```python
from build123d import *

# Parameters (mm, degrees)
SKETCH1_W               = 449.58
SKETCH1_H               = 449.58
BOSS_EXTRUDE1_DEPTH     = 6.35
CUT_EXTRUDE1_DEPTH      = 318.964480249
CUT_EXTRUDE1_DEPTH_BACK = 318.964480249
SKETCH2_R               = 1.984375
SKETCH2_R_2             = 27.432
SKETCH3_W               = 9.5
SKETCH3_H               = 12
CUT_EXTRUDE2_DEPTH      = 318.964480249
SKETCH4_R               = 2.1828125
CUT_EXTRUDE3_DEPTH      = 318.964480249
SKETCH5_R               = 2.1828125
CUT_EXTRUDE4_DEPTH      = 318.964480249


with BuildPart() as part:
    # Sketch1 → Boss-Extrude1 (new body)
    with BuildSketch(Plane(origin=(0, 0, 0), x_dir=(1, 0, 0), z_dir=(0, 1, 0))):
        Rectangle(SKETCH1_W, SKETCH1_H)
    extrude(amount=BOSS_EXTRUDE1_DEPTH)

    # Sketch2 → Cut-Extrude1 (cut, two sides: drawn at the far end of the back side and taken through both)
    with BuildSketch(Plane(origin=(0, 6.35, 0), x_dir=(1, 0, 0), z_dir=(0, 1, 0)).offset(-CUT_EXTRUDE1_DEPTH_BACK)):
        with Locations(Location((-44.8437, 44.8437, 0), (0, 0, 270))):
            Circle(SKETCH2_R)
        with Locations(Location((44.8437, 44.8437, 0), (0, 0, 270))):
            Circle(SKETCH2_R)
        with Locations(Location((-44.8437, -44.8437, 0), (0, 0, 270))):
            Circle(SKETCH2_R)
        with Locations(Location((44.8437, -44.8437, 0), (0, 0, 270))):
            Circle(SKETCH2_R)
        with Locations(Location((0, 0, 0), (0, 0, 270))):
            Circle(SKETCH2_R_2)
    extrude(amount=CUT_EXTRUDE1_DEPTH + CUT_EXTRUDE1_DEPTH_BACK, mode=Mode.SUBTRACT)

    # Sketch3 → Cut-Extrude2 (cut, through all)
    with BuildSketch(Plane(origin=(0, 6.35, 0), x_dir=(1, 0, 0), z_dir=(0, 1, 0))):
        with Locations((168.828815076, -168.828815076)):
            Rectangle(SKETCH3_W, SKETCH3_H)
    extrude(amount=-CUT_EXTRUDE2_DEPTH, mode=Mode.SUBTRACT)

    # Sketch4 → Cut-Extrude3 (cut, through all)
    with BuildSketch(Plane(origin=(0, 6.35, 0), x_dir=(1, 0, 0), z_dir=(0, 1, 0))):
        with Locations(Location((-212.09, 212.09, 0), (0, 0, 270))):
            Circle(SKETCH4_R)
        with Locations(Location((-186.69, 212.09, 0), (0, 0, 270))):
            Circle(SKETCH4_R)
        with Locations(Location((-212.09, 186.69, 0), (0, 0, 270))):
            Circle(SKETCH4_R)
        with Locations(Location((-186.69, 186.69, 0), (0, 0, 270))):
            Circle(SKETCH4_R)
        with Locations(Location((186.69, 212.09, 0), (0, 0, 270))):
            Circle(SKETCH4_R)
        with Locations(Location((186.69, 186.69, 0), (0, 0, 270))):
            Circle(SKETCH4_R)
        with Locations(Location((212.09, 186.69, 0), (0, 0, 270))):
            Circle(SKETCH4_R)
        with Locations(Location((212.09, 212.09, 0), (0, 0, 270))):
            Circle(SKETCH4_R)
        with Locations(Location((186.69, -186.69, 0), (0, 0, 270))):
            Circle(SKETCH4_R)
        with Locations(Location((212.09, -186.69, 0), (0, 0, 270))):
            Circle(SKETCH4_R)
        with Locations(Location((212.09, -212.09, 0), (0, 0, 270))):
            Circle(SKETCH4_R)
        with Locations(Location((186.69, -212.09, 0), (0, 0, 270))):
            Circle(SKETCH4_R)
        with Locations(Location((-212.09, -186.69, 0), (0, 0, 270))):
            Circle(SKETCH4_R)
        with Locations(Location((-186.69, -186.69, 0), (0, 0, 270))):
            Circle(SKETCH4_R)
        with Locations(Location((-186.69, -212.09, 0), (0, 0, 270))):
            Circle(SKETCH4_R)
        with Locations(Location((-212.09, -212.09, 0), (0, 0, 270))):
            Circle(SKETCH4_R)
    extrude(amount=-CUT_EXTRUDE3_DEPTH, mode=Mode.SUBTRACT)

    # Sketch5 → Cut-Extrude4 (cut, through all)
    with BuildSketch(Plane(origin=(0, 6.35, 0), x_dir=(1, 0, 0), z_dir=(0, 1, 0))):
        with Locations(Location((-191.419449709, 134.033341647, 0), (0, 0, 270))):
            Circle(SKETCH5_R)
        with BuildLine():
            ThreePointArc((-121.64596733, 192.580244977), (-139.176494703, 208.644013705), (-160.267293124, 219.623188433))
            ThreePointArc((-160.267293124, 219.623188433), (-163.065031767, 218.318581478), (-161.760424812, 215.520842836))
            ThreePointArc((-161.760424812, 215.520842836), (-141.680514333, 205.067903062), (-124.990230102, 189.774075318))
            ThreePointArc((-124.990230102, 189.774075318), (-121.915013887, 189.505028762), (-121.64596733, 192.580244977))
        make_face()
    extrude(amount=-CUT_EXTRUDE4_DEPTH, mode=Mode.SUBTRACT)


solid = part.part
```
The model under review builds one solid part; all positions refer to its coordinate system, in mm. Round coordinates to 2 decimals unless told otherwise and drop trailing zeros. Order: outer loops, then holes, each group sorted by start corner. A loop starts at its lowest first (then second) coordinate and runs counter-clockwise, first axis right, second up. Notation, with made-up numbers: (72.5, 8.25) - (84.5, 8.25) arc R12 ccw to (84.5, 30.25) - close; hole circle Ø2 at (18, 58.25). An arc over 180 degrees is marked (long way). Answer in a Markdown table with one row per item.
(1) Take a section at A-A on x = 0. Write out the cut boundary in (y, z).
Result set:
| item | result |
|---|---|
| outline | (0, -224.79) - (6.35, -224.79) - (6.35, -27.43) - (0, -27.43) - close; (0, 27.43) - (6.35, 27.43) - (6.35, 224.79) - (0, 224.79) - close |
(2) Mouldability with a two-part tool opening along X and no side actions: class faces 1 (the face through (-3, 0, -53)), 2 (the face through (-141.94, 3.22, -205.25)), 3 (the face through (-138.9, 3.22, -208.45)) as released by +X, released by -X, zero draft, split by the parting line, or undercut.
Result set:
| item | result |
|---|---|
| face 1 | zero draft |
| face 2 | undercut |
| face 3 | undercut |
(3) Take a section at B-B on z = 0. Write out the cut boundary in (x, y).
Result set:
| item | result |
|---|---|
| outline | (-224.79, 0) - (-27.43, 0) - (-27.43, 6.35) - (-224.79, 6.35) - close; (27.43, 0) - (224.79, 0) - (224.79, 6.35) - (27.43, 6.35) - close |
(4) For line 1 (Z direction, x = -186.69, y = 5); line 2 (Z direction, x = -137, y = 5.25), list the stretches that pass through material, from the lowest coordinate up. Write a range as from..to.
Result set:
| item | result |
|---|---|
| line 1 | z = -224.79..-214.27, -209.91..-188.87, -184.51..184.51, 188.87..209.91, 214.27..224.79 |
| line 2 | z = -224.79..-207.07, -201.55..224.79 |
(5) Clearance check with flat-ended pins moving along their axes: P1, Ø5, axis at x = 186.69, z = -212.09, coming from the +Y side; P2, Ø4, axis at x = 212.09, z = -186.69, coming from the -Y side. State where each tip first meets the part, or that it passes through.
Result set:
| item | result |
|---|---|
| P1 | stops at y = 6.35 |
| P2 | passes through |
